Could you check a few things on this model? Use its own coordinates, in mm. A direction names the side the tool comes from. Coordinates: 2 decimals unless noted, no trailing zeros. Loops run counter-clockwise (first coordinate to the right, second up) from the corner with the lowest first, then second, coordinate; pieces in that order, holes last. Notation, with made-up numbers: (81, 0.25) - (92, 0.25) arc R26 ccw to (92, 38.25) - close; hole circle Ø11 at (44, -23.75). An arc over 180 degrees is marked (long way). One line per item, written item: value. Start each with the question number.
(1) If we section it at B-B on x = -14.5: Write out the boundary of the cut face in (y, z) (3 decimals).
(2) On a 3-axis mill with a long thin cutter (end or side, diameter ignored), from which of +Z, -Z, +X, -X, +Y, -Y can I reach the whole of each face in a straight line? I mean faces 4 (the face through (-9.525, -2, 5)), 5 (the face through (-9.525, 34, 5)), 6 (the face through (-14, 35.175, 5)). Say none if no direction works.
(3) If we mould it in two halves opening along X, with no side actions, what happens to faces 1 (the face through (-7, 0, 5)), 2 (the face through (-5.001, 15.776, 6.576)), 3 (the face through (-1.432, 16.224, 8.167))? For each: pulls with the +X half, pulls with the -X half, needs draft (parallel to the pull), parting line crosses it, or undercut.
(4) If I drill on line 1 along Y through (x, z) = (-15.25, 4) (3 decimals); line 2 along Y through (x, z) = (-14.75, 6.75) (3 decimals); line 3 along Y through (x, z) = (-8.75, 7.5), over which ranges is the centre line in solid material (lowest first)? Write a range as from..to.
(5) I'm going to push flat-ended pins straight in: P1, Ø5, axis at x = -3.5, z = 5.5, coming from the -Y side; P2, Ø3.5, axis at y = -2, z = 7, coming from the +X side (3 decimals). Where does each tip first touch, or does it pass through?
(6) If we section it at A-A on y = 3.5: Count the separate pieces of the cut face and the enclosed holes in it, then the cut area to 3 significant figures.
```python
from build123d import *

# Parameters (mm, degrees)
F0_W     = 19.05
F0_H     = 32
F0_R     = 1.8288
F1_DEPTH = 9.525
F2_R     = 1.8288
F3_DEPTH = 32
F4_R     = 4.7625
F5_W     = 9.525
F5_H     = 3.175
F6_DEPTH = 9.525


with BuildPart() as f1:
    # F0 (on Top) → F1 (new body)
    with BuildSketch(Plane.XY):
        with Locations((-9.525, 16)):
            Rectangle(F0_W, F0_H)
        with Locations((-14.2875, 4.7625)):
            Circle(F0_R, mode=Mode.SUBTRACT)
        with Locations((-14.2875, 27.2375)):
            Circle(F0_R, mode=Mode.SUBTRACT)
    extrude(amount=F1_DEPTH)

    # F2 (on face) → F3 (cut, through all)
    with BuildSketch(Plane.XZ):
        with Locations((-4.7625, 4.7625)):
            Circle(F2_R)
    extrude(amount=-F3_DEPTH, mode=Mode.SUBTRACT)

    # F4
    f4_edges = [f1.edges().sort_by_distance(p)[0] for p in [
        (0, 16, 9.525),
    ]]
    fillet(f4_edges, radius=F4_R)

    # F5 (on face) → F6 (join, through all)
    with BuildSketch(Plane.XY.offset(9.525)):
        with Locations((-14.2875, 33.5875)):
            Rectangle(F5_W, F5_H)
        with Locations((-14.2875, -1.5875)):
            Rectangle(F5_W, F5_H)
    extrude(amount=-F6_DEPTH)


solid = f1.part
```
Values:
1. outline: (-3.175, 0) - (2.946, 0) - (2.946, 9.525) - (-3.175, 9.525) - close; (6.579, 0) - (25.421, 0) - (25.421, 9.525) - (6.579, 9.525) - close; (29.054, 0) - (35.175, 0) - (35.175, 9.525) - (29.054, 9.525) - close
2. face 4: +Z, -Z, +X, -Y
2. face 5: +Z, -Z, +X, +Y
2. face 6: +Z, -Z, +X, -X, +Y
3. face 1: needs draft
3. face 2: undercut
3. face 3: pulls with the +X half
4. line 1: y = -3.175..3.207, 6.318..25.682, 28.793..35.175
4. line 2: y = -3.175..2.993, 6.532..25.468, 29.007..35.175
4. line 3: y = 0..32
5. P1: stops at y = 0
5. P2: stops at x = -9.525
6. separate pieces: 2
6. enclosed holes: 1
6. area: 141 mm2
